CAD build for the part. Positions are in the model's coordinates, mm. A direction names the side the tool comes from. Coordinates: 2 decimals unless noted, no trailing zeros. Loops run counter-clockwise (first coordinate to the right, second up) from the corner with the lowest first, then second, coordinate; pieces in that order, holes last. Notation, with made-up numbers: (-1.5, -5.75) -> (40.5, -5.75) arc R16 cw to (40.5, 19.25) -> close; hole circle Ø2 at (88, 58). An arc over 180 degrees is marked (long way). Return JSON: item names as keys, results as strings. Group by question number.
(1) Saw through at B-B on y = -30. Write the cut outline in (x, z), then the cut area to 3 significant figures.
(2) Probe L1, parallel to Z at x = -39, y = -12; L2, parallel to X at y = -14.5, z = 24; L3, parallel to X at y = -37, z = -10.5. List the from-to ranges inside material, lowest first.
(3) Saw through at A-A on z = 4.5. Write the cut outline in (x, y), then the cut area to 3 significant figures.
(4) Tool access for faces 1 (the face through (-49.765, -25, 9)), 2 (the face through (-56.82, -1.8, 25.14)), 3 (the face through (-50.62, -49.1, 6.91)), 4 (the face through (-46.67, -25.34, -33.11)), 5 (the face through (-50.62, -0.9, 6.51)): list every direction of +Z, -Z, +X, -X, +Y, -Y with a clear straight run to the whole face (end or side of a thin tool).
(5) Saw through at C-C on x = -37. Write the cut outline in (y, z), then the cut area to 3 significant figures.
(6) Flat gauge pins, fed straight in: pin 1 Ø5 at (y, z) = (-6.5, 3.5) entering from +X; pin 2 Ø5 at (x, y) = (-52.5, -24) entering from +Z. Where does each tip first touch, or does it go through?
```python
from build123d import *

# Parameters (mm, degrees)
F1_DEPTH = 50
F2_R     = 6
F3_R     = 3


with BuildPart() as f1:
    # F0 (on Front) → F1 (new body)
    with BuildSketch(Plane.XZ):
        Polygon((-49.764752, 26.852785), (-63.764751, 26.852785), (-63.764751, -11.147215), (-46.805562, -33.426935), (-22.805792, -33.532045), (-22.744477, -19.532181), (-39.844699, -19.457288), (-49.764752, -6.42506), align=None)
    extrude(amount=F1_DEPTH)

    # F2
    f2_edges = [f1.edges().sort_by_distance(p)[0] for p in [
        (-56.764752, -50, 26.852785),
        (-56.764752, 0, 26.852785),
    ]]
    fillet(f2_edges, radius=F2_R)

    # F3
    f3_edges = [f1.edges().sort_by_distance(p)[0] for p in [
        (-63.764751, -25, -11.147215),
        (-63.764751, -50, 4.852785),
        (-55.285157, -50, -22.287075),
        (-44.804725, -50, -12.941174),
        (-49.764752, -50, 7.213862),
        (-46.805562, -25, -33.426935),
        (-55.285157, 0, -22.287075),
        (-44.804725, 0, -12.941174),
    ]]
    fillet(f3_edges, radius=F3_R)


solid = f1.part
```
Geometry results:
{
 "1": {"outline": "(-63.76, -10.14) arc R3 ccw to (-63.15, -11.95) -> (-47.7, -32.25) arc R3 ccw to (-45.33, -33.43) -> (-22.81, -33.53) -> (-22.74, -19.53) -> (-39.84, -19.46) -> (-49.76, -6.43) -> (-49.76, 23.85) arc R3 ccw to (-52.76, 26.85) -> (-60.76, 26.85) arc R3 ccw to (-63.76, 23.85) -> close", "area": "1,090 mm²"},
 "2": {"L1": "-33.46 to -19.46", "L2": "-63.76 to -49.77", "L3": "-63.74 to -46.66"},
 "3": {"outline": "(-63.76, -47) arc R3 ccw to (-60.76, -50) -> (-52.76, -50) arc R3 ccw to (-49.76, -47) -> (-49.76, -3) arc R3 ccw to (-52.76, 0) -> (-60.76, 0) arc R3 ccw to (-63.76, -3) -> close", "area": "692 mm²"},
 "4": {"face 1": "+Z, +X, +Y, -Y", "face 2": "+Z, +X, -X, +Y", "face 3": "+Z, +X, -Y", "face 4": "-Z, -X, +Y, -Y", "face 5": "+Z, +X, +Y"},
 "5": {"outline": "(-50, -33.47) -> (0, -33.47) -> (0, -19.47) -> (-50, -19.47) -> close", "area": "700 mm²"},
 "6": {"pin 1": "x = -49.76", "pin 2": "z = 26.85"}
}
